from build123d import *

# Parameters (mm, degrees)
SKETCH2_W           = 50
SKETCH2_H           = 300
BOSS_EXTRUDE1_DEPTH = 3.175
SKETCH3_R           = 1.025
SKETCH3_R_2         = 2.25
SKETCH3_W           = 29
SKETCH3_H           = 60
SKETCH3_W_2         = 19.62
SKETCH3_H_2         = 40.22
CUT_EXTRUDE1_DEPTH  = 6.35
CUT_EXTRUDE2_DEPTH  = 6.35
SKETCH5_R           = 3.175
SKETCH5_W           = 20
SKETCH5_H           = 90
CUT_EXTRUDE3_DEPTH  = 6.35


with BuildPart() as part:
    # Sketch2 → Boss-Extrude1 (new body)
    with BuildSketch(Plane(origin=(0, 0, 0), x_dir=(1, 0, 0), z_dir=(0, 1, 0))):
        with Locations((25, -150)):
            Rectangle(SKETCH2_W, SKETCH2_H)
    extrude(amount=BOSS_EXTRUDE1_DEPTH)

    # Sketch3 → Cut-Extrude1 (cut)
    with BuildSketch(Plane(origin=(0, 3.175, 0), x_dir=(1, 0, 0), z_dir=(0, 1, 0))):
        with Locations(Location((7.7, -21, 0), (0, 0, 270))):
            Circle(SKETCH3_R)
        with Locations(Location((7.7, -43, 0), (0, 0, 270))):
            Circle(SKETCH3_R)
        with Locations(Location((7.7, -65, 0), (0, 0, 270))):
            Circle(SKETCH3_R)
        with Locations(Location((42.3, -65, 0), (0, 0, 270))):
            Circle(SKETCH3_R)
        with Locations(Location((42.3, -43, 0), (0, 0, 270))):
            Circle(SKETCH3_R)
        with Locations(Location((42.3, -21, 0), (0, 0, 270))):
            Circle(SKETCH3_R)
        with Locations(Location((20, -291.07, 0), (0, 0, 270))):
            Circle(SKETCH3_R_2)
        with Locations(Location((30, -291.07, 0), (0, 0, 270))):
            Circle(SKETCH3_R_2)
        with Locations(Location((20, -242.39, 0), (0, 0, 270))):
            Circle(SKETCH3_R_2)
        with Locations(Location((30, -242.39, 0), (0, 0, 270))):
            Circle(SKETCH3_R_2)
        with Locations((25, -40.5)):
            Rectangle(SKETCH3_W, SKETCH3_H)
        with Locations((25, -266.73)):
            Rectangle(SKETCH3_W_2, SKETCH3_H_2)
    extrude(amount=-CUT_EXTRUDE1_DEPTH, mode=Mode.SUBTRACT)

    # Sketch4 → Cut-Extrude2 (cut)
    with BuildSketch(Plane(origin=(0, 3.175, 0), x_dir=(1, 0, 0), z_dir=(0, 1, 0))):
        with BuildLine():
            Line((0, 0), (0, -25))
            ThreePointArc((0, -25), (7.32233047, -7.32233047), (25, 0))
            Line((25, 0), (0, 0))
        make_face()
        with BuildLine():
            ThreePointArc((25, 0), (42.67766953, -7.32233047), (50, -25))
            Line((50, -25), (50, 0))
            Line((50, 0), (25, 0))
        make_face()
        with BuildLine():
            ThreePointArc((25, -300), (7.32233047, -292.67766953), (0, -275))
            Line((0, -275), (0, -300))
            Line((0, -300), (25, -300))
        make_face()
        with BuildLine():
            Line((50, -300), (50, -275))
            ThreePointArc((50, -275), (42.67766953, -292.67766953), (25, -300))
            Line((25, -300), (50, -300))
        make_face()
    extrude(amount=-CUT_EXTRUDE2_DEPTH, mode=Mode.SUBTRACT)

    # Sketch5 → Cut-Extrude3 (cut)
    with BuildSketch(Plane.XZ):
        with Locations(Location((25, 215, 0), (0, 0, 270))):
            Circle(SKETCH5_R)
        with Locations(Location((25, 85, 0), (0, 0, 90))):
            Circle(SKETCH5_R)
        with Locations((25, 150)):
            Rectangle(SKETCH5_W, SKETCH5_H)
    extrude(amount=-CUT_EXTRUDE3_DEPTH, mode=Mode.SUBTRACT)


solid = part.part
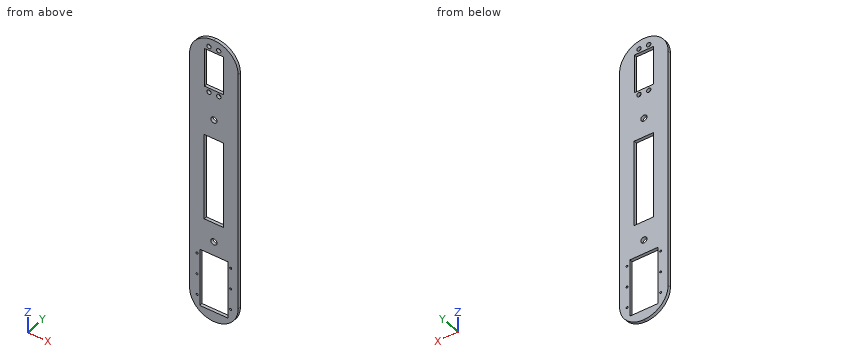
Here's how the part is built. I have some questions about the finished solid (model axes, mm). Round coordinates to 2 decimals unless told otherwise and drop trailing zeros. Order: outer loops, then holes, each group sorted by start corner. A loop starts at its lowest first (then second) coordinate and runs counter-clockwise, first axis right, second up. Notation, with made-up numbers: M 54.5,62 L 76.5,62 A21 ccw 76.5,100 Z; hole C -1,7.25 d10. An arc over 180 degrees is marked long. Return JSON: item names as keys, results as strings. Group by question number.
1. Please list where these lines run through material, in increasing order: probe 1 along X at (y, z) = (1.4, 43) (3 decimals); probe 2 along X at (y, z) = (2.95, 122.5); probe 3 along X at (y, z) = (0.9, 291.07).
2. If we section it at A-A on z = 257: List the corners of the cut face in (x, y) for me (3 decimals), then the cut area to 3 significant figures.
3. If we section it at B-B on y = 1.3: State how many separate pieces and enclosed holes the cut face has, then the cut area to 3 significant figures.
4. If we section it at C-C on z = 85: List the corners of the cut face in (x, y) for me (3 decimals), then the cut area to 3 significant figures.
5. I'm going to push flat-ended pins straight in: pin 1 Ø1 at (x, y) = (26.5, 2) entering from +Z; pin 2 Ø1.5 at (x, y) = (34, 1.5) entering from +Z; pin 3 Ø1.5 at (x, y) = (26.5, 2.5) entering from -Z. Where does each tip first touch, or does it pass through?
6. If we section it at D-D on x = 47: List the corners of the cut face in (y, z) for me (3 decimals), then the cut area to 3 significant figures.
Reply:
{
 "1": {"probe 1": "0 to 6.675, 8.725 to 10.5, 39.5 to 41.275, 43.325 to 50", "probe 2": "0 to 15, 35 to 50", "probe 3": "5.85 to 17.75, 22.25 to 27.75, 32.25 to 44.15"},
 "2": {"outline": "M 0,0 L 15.19,0 L 15.19,3.175 L 0,3.175 Z; M 34.81,0 L 50,0 L 50,3.175 L 34.81,3.175 Z", "area": "96.5 mm^2"},
 "3": {"separate pieces": "1", "enclosed holes": "15", "area": "9,990 mm^2"},
 "4": {"outline": "M 0,0 L 21.825,0 L 21.825,3.175 L 0,3.175 Z; M 28.175,0 L 50,0 L 50,3.175 L 28.175,3.175 Z", "area": "139 mm^2"},
 "5": {"pin 1": "z = 299.98", "pin 2": "z = 298.6", "pin 3": "z = 0.01"},
 "6": {"outline": "M 0,13.126 L 3.175,13.126 L 3.175,286.874 L 0,286.874 Z", "area": "869 mm^2"}
}
